Source: CAD feature listing. Evaluate the final solid. Frame: model axes, mm. A direction names the side the tool comes from. Coordinates: 2 decimals unless noted, no trailing zeros. Loops run counter-clockwise (first coordinate to the right, second up) from the corner with the lowest first, then second, coordinate; pieces in that order, holes last. Notation, with made-up numbers: M 54,30 L 82,30 A11 cw 82,40 Z; hole C 52.5,-15.75 d8. An arc over 180 degrees is marked long. One line per question, with ' | ' between items. Start each with the question number.
1. Section query A-A, the plane x = 4.5. Output: boundary loops of the cut face in (y, z), and give its area (3 significant figures).
2. Ray query, probe 1 along Y at (x, z) = (55.5, 1.25); probe 2 along X at (y, z) = (-75.5, 0.5); probe 3 along Z at (x, y) = (49, -61.5). Return the intervals inside material, ascending.
3. Access query for faces 4 (the flat face through (34.5, -40, 6)), 5 (the flat face through (25.5, -40, 6)), 6 (the cylindrical face through (26.1, -43.93, 6.57)). Directions: +Z, -Z, +X, -X, +Y, -Y. A direction counts if a zero-diameter tool reaches every point of the face in a straight line with its end or side. Return the directions, or none.
4. Section query C-C, the plane z = 7.75. Output: boundary loops of the cut face in (x, y).
5. Section query D-D, the plane y = -34. Output: boundary loops of the cut face in (x, z).
6. Pin query (flat end, axial travel): P1, Ø3, axis at x = 4.5, y = -4.5, coming from the -Z side; P2, Ø2.5, axis at x = 29, z = 8, coming from the +Y side; P3, Ø1.5, axis at y = -40.5, z = 4.5, coming from the -X side; P4, Ø4, axis at x = 28.5, z = 8, coming from the -Y side. Return the tip coordinate at first contact, or that it passes through.
7. Mould query, pull axis Y, two halves, no side actions, for faces 1 (the flat face through (30, -39, 0)), 2 (the cylindrical face through (59.4, -79.43, 1.01)), 3 (the cylindrical face through (57.026, -4.019, 0.76)). Classes: pulls with the +Y half, pulls with the -Y half, needs draft (parallel to the pull), parting line crosses it, or undercut.
8. Section query B-B, the plane y = -4.5. Output: boundary loops of the cut face in (x, z).
```python
from build123d import *

# Parameters (mm, degrees)
SKETCH_W        = 60
SKETCH_H        = 80
PAD_DEPTH       = 1.5
SKETCH001_R     = 1.6
POCKET_DEPTH    = 5
SKETCH002_W     = 9
SKETCH002_H     = 9
PAD001_DEPTH    = 11
FILLET_R        = 2
CHAMFER_SIZE    = 1
FILLET001_R     = 2
CHAMFER001_SIZE = 0.5


with BuildPart() as part:
    # Sketch → Pad (new body)
    with BuildSketch(Plane.XY):
        with Locations((30, -40)):
            Rectangle(SKETCH_W, SKETCH_H)
    extrude(amount=PAD_DEPTH)

    # Sketch001 (on Face6 of Pad) → Pocket (cut)
    with BuildSketch(Plane.XY.offset(1.5)):
        with Locations((4.5, -4.5)):
            Circle(SKETCH001_R)
        with Locations((55.5, -4.5)):
            Circle(SKETCH001_R)
        with Locations((4.5, -75.5)):
            Circle(SKETCH001_R)
        with Locations((55.5, -75.5)):
            Circle(SKETCH001_R)
    extrude(amount=-POCKET_DEPTH, mode=Mode.SUBTRACT)

    # Sketch002 (on Face5 of Pocket) → Pad001 (join)
    with BuildSketch(Plane.XY.offset(1.5)):
        with Locations((30, -40)):
            Rectangle(SKETCH002_W, SKETCH002_H)
    extrude(amount=PAD001_DEPTH)

    # Fillet
    fillet_edges = [part.edges().sort_by_distance(p)[0] for p in [
        (25.5, -44.5, 7),
        (34.5, -44.5, 7),
        (34.5, -35.5, 7),
        (25.5, -35.5, 7),
    ]]
    fillet(fillet_edges, radius=FILLET_R)

    # Chamfer
    chamfer_edges = [part.edges().sort_by_distance(p)[0] for p in [
        (30, -44.5, 12.5),
    ]]
    chamfer(chamfer_edges, length=CHAMFER_SIZE)

    # Fillet001
    fillet001_edges = [part.edges().sort_by_distance(p)[0] for p in [
        (0, -80, 0.75),
        (60, -80, 0.75),
        (60, 0, 0.75),
        (0, 0, 0.75),
    ]]
    fillet(fillet001_edges, radius=FILLET001_R)

    # Chamfer001
    chamfer001_edges = [part.edges().sort_by_distance(p)[0] for p in [
        (30, 0, 0),
    ]]
    chamfer(chamfer001_edges, length=CHAMFER001_SIZE)


solid = part.part
```
Taken from the geometry:
1) outline: M -80,0.5 L -79.5,0 L -77.1,0 L -77.1,1.5 L -80,1.5 Z; M -73.9,0 L -6.1,0 L -6.1,1.5 L -73.9,1.5 Z; M -2.9,0 L -0.5,0 L 0,0.5 L 0,1.5 L -2.9,1.5 Z | area: 110 mm^2
2) probe 1: -80 to -77.1, -73.9 to -6.1, -2.9 to 0 | probe 2: 0 to 2.9, 6.1 to 53.9, 57.1 to 60 | probe 3: 0 to 1.5
3) face 4: +Z, +X, +Y, -Y | face 5: +Z, -X, +Y, -Y | face 6: +Z, -X, -Y
4) outline: M 25.5,-42.5 A2 ccw 27.5,-44.5 L 32.5,-44.5 A2 ccw 34.5,-42.5 L 34.5,-37.5 A2 ccw 32.5,-35.5 L 27.5,-35.5 A2 ccw 25.5,-37.5 Z
5) outline: M 0,0.5 L 0.5,0 L 59.5,0 L 60,0.5 L 60,1.5 L 0,1.5 Z
6) P1: through | P2: y = -35.5 | P3: x = 25.5 | P4: y = -44.5
7) face 1: needs draft | face 2: pulls with the -Y half | face 3: undercut
8) outline: M 0,0.5 L 0.5,0 L 2.9,0 L 2.9,1.5 L 0,1.5 Z; M 6.1,0 L 53.9,0 L 53.9,1.5 L 6.1,1.5 Z; M 57.1,0 L 59.5,0 L 60,0.5 L 60,1.5 L 57.1,1.5 Z
